Geometry check sheet. Reference: the model listing, model coordinates, mm. Give positions to 0.01 mm unless a question says otherwise; leave off trailing zeros. Write each loop counter-clockwise with the first axis right and the second up, starting at its lowest first coordinate (ties: lowest second). Pieces come first, ordered by that corner, then holes. Notation, with made-up numbers: (-37, -34) -> (-10, -34) arc R22 ccw to (-10, -19) -> close; hole circle Ø2 at (-15, 32.25). An arc over 180 degrees is marked (long way). One line per item, written item: value.
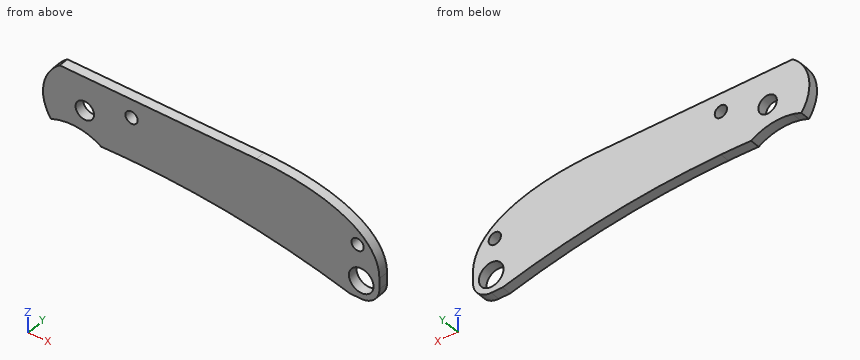
from build123d import *

# Parameters (mm, degrees)
F0_W      = 82.55
F0_H      = 23.368
F0_R      = 2.38125
F1_DEPTH  = 2.54
F2_R      = 1.5875
F3_DEPTH  = 12.7
F5_DEPTH  = 2.541
F7_DEPTH  = 2.5410001
F8_R      = 4.699
F10_DEPTH = 2.54
F11_R     = 3.175
F11_R_2   = 1.5875
F12_DEPTH = 2.5410001


with BuildPart() as f1:
    # F0 (on Front) → F1 (new body)
    with BuildSketch(Plane.XZ):
        with Locations((34.798, -3.048)):
            Rectangle(F0_W, F0_H)
        Circle(F0_R, mode=Mode.SUBTRACT)
    extrude(amount=F1_DEPTH)

    # F2 (on face) → F3 (cut, symmetric)
    with BuildSketch(Plane.XZ.offset(2.54)):
        with Locations((12.065, 3.937)):
            Circle(F2_R)
    extrude(amount=F3_DEPTH, both=True, mode=Mode.SUBTRACT)

    # F4 (on face) → F5 (cut, through all)
    with BuildSketch(Plane.XZ.offset(2.54)):
        with BuildLine():
            ThreePointArc((68.453, -14.732), (40.5068335951, -9.1204471828), (12.065, -7.239))
            ThreePointArc((12.065, -7.239), (2.7854261498, -7.4384974289), (-6.477, -8.0366210649))
            Line((-6.477, -8.0366210649), (-6.477, -14.732))
            Line((-6.477, -14.732), (68.453, -14.732))
        make_face()
        with BuildLine():
            add(Edge.make_bspline(
                [(76.073, -7.239), (76.073, 8.636), (44.323, 8.636)],
                knots=[6.1622777964, 6.1622777964, 6.1622777964, 7.2142515659, 7.2142515659, 7.2142515659], degree=2, weights=[1, 0.8648288808, 1]))
            Line((76.073, -7.239), (76.073, 8.636))
            Line((76.073, 8.636), (44.323, 8.636))
        make_face()
    extrude(amount=-F5_DEPTH, mode=Mode.SUBTRACT)

    # F6 (on face) → F7 (cut, through all)
    with BuildSketch(Plane.XZ.offset(2.54)):
        with BuildLine():
            Line((-12.7, -9.017), (6.35, -9.017))
            ThreePointArc((6.35, -9.017), (-3.175, -5.207), (-12.7, -9.017))
        make_face()
    extrude(amount=-F7_DEPTH, mode=Mode.SUBTRACT)

    # F8
    f8_edges = [f1.edges().sort_by_distance(p)[0] for p in [
        (76.073, -1.27, -14.732),
    ]]
    fillet(f8_edges, radius=F8_R)

    # F9 (on face) → F10 (join)
    with BuildSketch(Plane.XZ.offset(2.54)):
        with BuildLine():
            Line((-6.477, -5.6075295659), (-6.477, 8.636))
            ThreePointArc((-6.477, 8.636), (-10.6766730669, 1.5939501943), (-8.7169373329, -6.3676548693))
            ThreePointArc((-8.7169373329, -6.3676548693), (-7.6132715674, -5.9395508271), (-6.477, -5.6075295659))
        make_face()
    extrude(amount=-F10_DEPTH)

    # F11 (on face) → F12 (cut, through all)
    with BuildSketch(Plane.XZ.offset(2.54)):
        with Locations((71.374, -10.033)):
            Circle(F11_R)
        with Locations((70.4395100474, -1.0937360348)):
            Circle(F11_R_2)
    extrude(amount=-F12_DEPTH, mode=Mode.SUBTRACT)


solid = f1.part
1) Sectioned sample at B-B on x = 23.5. Record the cut outline in (y, z).
Verdict:
outline: (-2.54, -7.54) -> (0, -7.54) -> (0, 8.64) -> (-2.54, 8.64) -> close
2) Sectioned sample at C-C on y = -2.1. Give the number of separate pieces and of enclosed holes in the cut face, plus the area to 3 significant figures.
Verdict:
separate pieces: 1
enclosed holes: 4
area: 1,380 mm^2
3) Depth check by flat-ended pin: pin 1 Ø1.9 at (x, z) = (12.065, 3.937) entering from -Y. Enter the tip coordinate at first touch or a pass-through.
Verdict:
pin 1: through
4) Sectioned sample at A-A on x = 0. Record the cut outline in (y, z), plus the area to 3 significant figures.
Verdict:
outline: (-2.54, -5.58) -> (0, -5.58) -> (0, -2.38) -> (-2.54, -2.38) -> close; (-2.54, 2.38) -> (0, 2.38) -> (0, 8.64) -> (-2.54, 8.64) -> close
area: 24.0 mm^2
5) Sectioned sample at D-D on x = 37. Record the cut outline in (y, z).
Verdict:
outline: (-2.54, -8.68) -> (0, -8.68) -> (0, 8.64) -> (-2.54, 8.64) -> close
6) Scan lines: probe 1 along Z at (x, y) = (71.5, -1.65); probe 2 along Z at (x, y) = (11.5, -1.25); probe 3 along Z at (x, y) = (0, -1.45). Record each from-to range of solid material in increasing order.
Verdict:
probe 1: -14.73 to -13.21, -6.86 to -2.28, 0.09 to 1.86
probe 2: -7.24 to 2.45, 5.42 to 8.64
probe 3: -5.58 to -2.38, 2.38 to 8.64
